from build123d import *

# Parameters (mm, degrees)
SKETCH1_W           = 304.8
SKETCH1_H           = 63.5
SKETCH1_R           = 19.05
BOSS_EXTRUDE1_DEPTH = 6.35


with BuildPart() as part:
    # Sketch1 → Boss-Extrude1 (new body)
    # profile 1 of 3: a face of its own
    with BuildSketch(Plane(origin=(0, 0, 0), x_dir=(1, 0, 0), z_dir=(0, 1, 0))):
        with Locations((152.4, 31.75)):
            Rectangle(SKETCH1_W, SKETCH1_H)
        with Locations((152.4, 31.75)):
            Circle(SKETCH1_R, mode=Mode.SUBTRACT)
    # profile 2 of 3: a face of its own
    with BuildSketch(Plane(origin=(0, 0, 0), x_dir=(1, 0, 0), z_dir=(0, 1, 0))):
        with BuildLine():
            Line((138.929615818, 45.220384182), (165.870384182, 45.220384182))
            ThreePointArc((165.870384182, 45.220384182), (152.4, 50.8), (138.929615818, 45.220384182))
        make_face()
    # profile 3 of 3: a face of its own
    with BuildSketch(Plane(origin=(0, 0, 0), x_dir=(1, 0, 0), z_dir=(0, 1, 0))):
        with BuildLine():
            ThreePointArc((138.929615818, 18.279615818), (152.4, 12.7), (165.870384182, 18.279615818))
            Line((165.870384182, 18.279615818), (138.929615818, 18.279615818))
        make_face()
    extrude(amount=BOSS_EXTRUDE1_DEPTH)


solid = part.part
The listing builds one solid part. Answer for the finished solid, in the listing's coordinates (mm). A direction names the side the tool comes from. Give positions to 0.01 mm unless a question says otherwise; leave off trailing zeros. Loops run counter-clockwise (first coordinate to the right, second up) from the corner with the lowest first, then second, coordinate; pieces in that order, holes last. Notation, with made-up numbers: (-9.5, 33) - (47.5, 33) arc R15 ccw to (47.5, 53) - close; hole circle Ø7 at (52, -27). An arc over 180 degrees is marked (long way). Write each question's results on one line, items separated by ' | '.
1. Find section A-A, the plane y = 3. Write down the section's boundary in (x, z), then the cut area to 3 significant figures.
Resolved:
outline: (0, -63.5) - (304.8, -63.5) - (304.8, 0) - (0, 0) - close; hole (138.93, -45.22) - (165.87, -45.22) arc R19.05 ccw to (165.87, -18.28) - (138.93, -18.28) arc R19.05 ccw to start | area: 18,400 mm^2
2. Consider probe 1 along Z at (x, y) = (150.5, 1.5); probe 2 along X at (y, z) = (1, -32); probe 3 along Z at (x, y) = (136, 1). Determine where each line is inside the solid, lowest interval first. Write a range as from..to.
Resolved:
probe 1: z = -63.5..-45.22, -18.28..0 | probe 2: x = 0..133.35, 171.45..304.8 | probe 3: z = -63.5..-41.44, -22.06..0
3. Find section B-B, the plane z = -26.5. Write down the section's boundary in (x, y), then the cut area to 3 significant figures.
Resolved:
outline: (0, 0) - (134.09, 0) - (134.09, 6.35) - (0, 6.35) - close; (170.71, 0) - (304.8, 0) - (304.8, 6.35) - (170.71, 6.35) - close | area: 1,700 mm^2
4. For a pull along X with two mould halves and no side action, classify faces 3 (the face through (304.8, 3, -31)), 4 (the face through (152, 3, -45.22)), 5 (the face through (150, 6.35, -18)) as +X half, -X half, draft (parallel to the pull), parting line (faces both ways), or undercut.
Resolved:
face 3: +X half | face 4: undercut | face 5: draft
5. Which of the six approach directions +Z, -Z, +X, -X, +Y, -Y give full straight-line access (tool end or side, diameter ignored) to faces 1 (the face through (171.45, 3.13, -31.54)), 2 (the face through (0, 3, -31))?
Resolved:
face 1: +Y, -Y | face 2: +Z, -Z, -X, +Y, -Y
6. A flat-ended cylindrical pin translates along its axis: P1, Ø8, axis at x = 143.5, z = -25.5, coming from the +Y side. Find the tip coordinate at first contact, or state that the pin passes through.
Resolved:
P1: passes through
